from build123d import *

# Parameters (mm, degrees)
SKETCH1_W               = 50.8
SKETCH1_H               = 50.8
SKETCH1_W_2             = 47.625
SKETCH1_H_2             = 47.625
BOSS_EXTRUDE1_DEPTH     = 254
SKETCH4_R               = 2.3999952
CUT_EXTRUDE1_DEPTH      = 50.2125
CUT_EXTRUDE1_DEPTH_BACK = 2.5875
SKETCH5_R               = 2.3999952
CUT_EXTRUDE2_DEPTH      = 51.8
SKETCH6_R               = 2.3999952
CUT_EXTRUDE3_DEPTH      = 1
CUT_EXTRUDE3_DEPTH_BACK = 51.8
SKETCH7_R               = 2.3999952
CUT_EXTRUDE4_DEPTH      = 1
CUT_EXTRUDE4_DEPTH_BACK = 51.8
SKETCH8_R               = 3.175
CUT_EXTRUDE5_DEPTH      = 1
CUT_EXTRUDE5_DEPTH_BACK = 51.8
SKETCH9_R               = 3.175
CUT_EXTRUDE6_DEPTH      = 1
CUT_EXTRUDE6_DEPTH_BACK = 51.8
SKETCH10_W              = 24.13
SKETCH10_H              = 25.4
CUT_EXTRUDE7_DEPTH      = 24.13


with BuildPart() as part:
    # Sketch1 → Boss-Extrude1 (new body)
    with BuildSketch(Plane(origin=(0, 0, 0), x_dir=(1, 0, 0), z_dir=(0, 1, 0))):
        Rectangle(SKETCH1_W, SKETCH1_H)
        Rectangle(SKETCH1_W_2, SKETCH1_H_2, mode=Mode.SUBTRACT)
    extrude(amount=BOSS_EXTRUDE1_DEPTH)

    # Sketch4 → Cut-Extrude1 (cut, two sides)
    with BuildSketch(Plane(origin=(-23.8125, 0, 0), x_dir=(0, 0, -1), z_dir=(1, 0, 0))) as cut_extrude1_sk:
        with Locations((0, 241.587599882)):
            Circle(SKETCH4_R)
    extrude(amount=CUT_EXTRUDE1_DEPTH, mode=Mode.SUBTRACT)
    extrude(cut_extrude1_sk.sketch, amount=-CUT_EXTRUDE1_DEPTH_BACK, mode=Mode.SUBTRACT)

    # Sketch5 → Cut-Extrude2 (cut, through all)
    with BuildSketch(Plane(origin=(0, 0, -25.4), x_dir=(-1, 0, 0), z_dir=(0, 0, -1))):
        with Locations((0, 241.587599882)):
            Circle(SKETCH5_R)
    extrude(amount=-CUT_EXTRUDE2_DEPTH, mode=Mode.SUBTRACT)

    # Sketch6 → Cut-Extrude3 (cut, two sides)
    with BuildSketch(Plane(origin=(25.4, 0, 0), x_dir=(0, 0, -1), z_dir=(1, 0, 0))) as cut_extrude3_sk:
        with Locations((0, 12.412400118)):
            Circle(SKETCH6_R)
    extrude(amount=CUT_EXTRUDE3_DEPTH, mode=Mode.SUBTRACT)
    extrude(cut_extrude3_sk.sketch, amount=-CUT_EXTRUDE3_DEPTH_BACK, mode=Mode.SUBTRACT)

    # Sketch7 → Cut-Extrude4 (cut, two sides)
    with BuildSketch(Plane(origin=(0, 0, -25.4), x_dir=(-1, 0, 0), z_dir=(0, 0, -1))) as cut_extrude4_sk:
        with Locations((0, 12.412400118)):
            Circle(SKETCH7_R)
    extrude(amount=CUT_EXTRUDE4_DEPTH, mode=Mode.SUBTRACT)
    extrude(cut_extrude4_sk.sketch, amount=-CUT_EXTRUDE4_DEPTH_BACK, mode=Mode.SUBTRACT)

    # Sketch8 → Cut-Extrude5 (cut, two sides)
    with BuildSketch(Plane(origin=(0, 0, -25.4), x_dir=(-1, 0, 0), z_dir=(0, 0, -1))) as cut_extrude5_sk:
        with Locations((0, 228.6)):
            Circle(SKETCH8_R)
    extrude(amount=CUT_EXTRUDE5_DEPTH, mode=Mode.SUBTRACT)
    extrude(cut_extrude5_sk.sketch, amount=-CUT_EXTRUDE5_DEPTH_BACK, mode=Mode.SUBTRACT)

    # Sketch9 → Cut-Extrude6 (cut, two sides)
    with BuildSketch(Plane(origin=(25.4, 0, 0), x_dir=(0, 0, -1), z_dir=(1, 0, 0))) as cut_extrude6_sk:
        with Locations((0, 228.6)):
            Circle(SKETCH9_R)
    extrude(amount=CUT_EXTRUDE6_DEPTH, mode=Mode.SUBTRACT)
    extrude(cut_extrude6_sk.sketch, amount=-CUT_EXTRUDE6_DEPTH_BACK, mode=Mode.SUBTRACT)

    # Sketch10 → Cut-Extrude7 (cut)
    with BuildSketch(Plane(origin=(25.4, 0, 0), x_dir=(0, 0, -1), z_dir=(1, 0, 0))):
        with Locations((-13.335, 190.5)):
            Rectangle(SKETCH10_W, SKETCH10_H)
    extrude(amount=-CUT_EXTRUDE7_DEPTH, mode=Mode.SUBTRACT)


solid = part.part
Could you check a few things on this model? Use its own coordinates, in mm. A direction names the side the tool comes from. Give positions to 0.01 mm unless a question says otherwise; leave off trailing zeros. Order: outer loops, then holes, each group sorted by start corner. A loop starts at its lowest first (then second) coordinate and runs counter-clockwise, first axis right, second up.
1. Suppose I cut it at D-D (x = -12). List the corners of the cut face in (y, z) for me, plus the area to 3 significant figures.
2. Suppose I cut it at C-C (y = 228.6). List the corners of the cut face in (x, z) for me (1 decimal), plus the area to 3 significant figures.
3. Will these pins go through, and if not, where does the flat tip stop? P1, Ø3, axis at y = 12.41, z = 0, coming from the -X side; P2, Ø1.7, axis at x = 24.5, y = 190, coming from the +Z side; P3, Ø7.5, axis at x = 0, y = 228.6, coming from the -Z side.
4. For faces 5 (the flat face through (0, 125, 25.4)), 6 (the flat face through (0, 125, 23.812)), 7 (the flat face through (19, 203.2, 24)), which set-ups out of +Z, -Z, +X, -X, +Y, -Y let a thin tool reach every point of the face, with its end or its side?
5. Suppose I cut it at A-A (x = 20). List the corners of the cut face in (y, z) for me.
6. Suppose I cut it at B-B (z = 8). List the corners of the cut face in (x, y) for me.
7. We'd pull the mould along Y, two halves only. Please class faces 1 (the flat face through (-2, 254, 24)), 2 (the flat face through (19, 177.8, 24)), 3 (the flat face through (-23.812, 125, 0)), 4 (the flat face through (-2, 0, 24)): pulls with the +Y half, pulls with the -Y half, needs draft (parallel to the pull), parting line crosses it, or undercut.
8. I need wall thicknesses on L1, parallel to Y at x = 25.05, z = 0 (3 decimals); L2, parallel to Z at x = 7, y = 147. Which ranges of each line are inside material? Lowest first, please.
Solved:
1. outline: (0, -25.4) - (254, -25.4) - (254, -23.81) - (0, -23.81) - close; (0, 23.81) - (254, 23.81) - (254, 25.4) - (0, 25.4) - close
1. area: 806 mm2
2. outline: (-25.4, -25.4) - (-3.2, -25.4) - (-3.2, -23.8) - (-23.8, -23.8) - (-23.8, -3.2) - (-25.4, -3.2) - close; (-25.4, 3.2) - (-23.8, 3.2) - (-23.8, 23.8) - (-3.2, 23.8) - (-3.2, 25.4) - (-25.4, 25.4) - close; (3.2, -25.4) - (25.4, -25.4) - (25.4, -3.2) - (23.8, -3.2) - (23.8, -23.8) - (3.2, -23.8) - close; (3.2, 23.8) - (23.8, 23.8) - (23.8, 3.2) - (25.4, 3.2) - (25.4, 25.4) - (3.2, 25.4) - close
2. area: 272 mm2
3. P1: passes through
3. P2: stops at z = 1.27
3. P3: stops at z = -25.4
4. face 5: +Z, +X, -X, +Y, -Y
4. face 6: +Y, -Y
4. face 7: +Z, +X
5. outline: (0, -25.4) - (254, -25.4) - (254, -23.81) - (0, -23.81) - close; (0, 23.81) - (177.8, 23.81) - (177.8, 25.4) - (0, 25.4) - close; (203.2, 23.81) - (254, 23.81) - (254, 25.4) - (203.2, 25.4) - close
6. outline: (-25.4, 0) - (-23.81, 0) - (-23.81, 254) - (-25.4, 254) - close; (23.81, 0) - (25.4, 0) - (25.4, 177.8) - (23.81, 177.8) - close; (23.81, 203.2) - (25.4, 203.2) - (25.4, 254) - (23.81, 254) - close
7. face 1: pulls with the +Y half
7. face 2: undercut
7. face 3: needs draft
7. face 4: pulls with the -Y half
8. L1: y = 0 to 10.012, 14.812 to 225.425, 231.775 to 239.188, 243.988 to 254
8. L2: z = -25.4 to -23.81, 23.81 to 25.4
